Design review of the part built by this model. Coordinates are the model's own, in mm. A direction names the side the tool comes from. Coordinates: 2 decimals unless noted, no trailing zeros. Write each loop counter-clockwise with the first axis right and the second up, starting at its lowest first coordinate (ties: lowest second). Pieces come first, ordered by that corner, then holes. Notation, with made-up numbers: (54, 10.25) - (74, 10.25) arc R20 cw to (74, 18.25) - close; hole circle Ø7 at (-16.75, 26.25). An arc over 180 degrees is marked (long way). Answer as CSV lines item,"result". Start each with the question number.
Q1. We need section B-B (y = 2.4). Write out the cut boundary in (x, z).
Q2. We need section A-A (x = -6.35). Write out the cut boundary in (y, z) (3 decimals), plus the area to 3 significant figures.
Q3. Mouldability with a two-part tool opening along X and no side actions: class faces 5 (the face through (0, 2, -8)), 6 (the face through (52.003, 1.565, -51.522)), 7 (the face through (22, 2, -6.537)) as pulls with the +X half, pulls with the -X half, needs draft (parallel to the pull), parting line crosses it, or undercut.
Q4. For line 1 along Z through (x, y) = (50.8, 2.3); line 2 along X through (y, z) = (2.1, -50); line 3 along Z through (x, y) = (48, 0.7), list the stretches that pass through material, from the lowest coordinate up. Write a range as [from, to].
Q5. We need section C-C (z = -36). Write out the cut boundary in (x, y) (3 decimals), plus the area to 3 significant figures.
Q6. Machinability: for faces 1 (the face through (44.45, 2, -9)), 2 (the face through (54, 2, -29.464)), 3 (the face through (-9, 2, -10.414)), 4 (the face through (0, 2, -35)), which of the approach directions +Z, -Z, +X, -X, +Y, -Y give a long, thin tool a straight path to every point of the face, cutting with its end or side? Answer none if there is none.
Q7. Clearance check with flat-ended pins moving along their axes: pin 1 (2 mm diameter, centred on x = 50.8, z = -50.419, fed in from +Y); pin 2 (1 mm diameter, centred on x = 56, y = 1.5, fed in from +Z); pin 3 (8 mm diameter, centred on x = 39, z = -22.5, fed in from -Y); pin 4 (1 mm diameter, centred on y = 1.5, z = -37.5, fed in from -X). State where each tip first meets the part, or that it passes through.
from build123d import *

# Parameters (mm, degrees)
BOSS_EXTRUDE1_DEPTH   = 3.175
F_4_CLEARANCE_HOLE1_D = 3.2639
SKETCH6_W             = 47.36250333
SKETCH6_H             = 20.126599321
CUT_EXTRUDE2_DEPTH    = 95.829208522
SKETCH8_W             = 57.220052793
SKETCH8_H             = 21.750209978
CUT_EXTRUDE4_DEPTH    = 88.381999067


with BuildPart() as part:
    # Sketch2 → Boss-Extrude1 (new body)
    with BuildSketch(Plane(origin=(0, 0, 0), x_dir=(1, 0, 0), z_dir=(0, 1, 0))):
        Polygon((0, 40.894), (-19.05, 40.894), (-19.05, 59.944), (0, 59.944), (0, 70.358), (44.45, 70.358), (44.45, 59.944), (63.5, 59.944), (63.5, 40.894), (44.45, 40.894), (44.45, 29.464), (63.5, 29.464), (63.5, 10.414), (44.45, 10.414), (44.45, 0), (0, 0), (0, 10.414), (-19.05, 10.414), (-19.05, 29.464), (0, 29.464), align=None)
    extrude(amount=BOSS_EXTRUDE1_DEPTH)

    # #4 Clearance Hole1 (through all)
    with Locations(Plane(origin=(0, 3.175, 0), x_dir=(1, 0, 0), z_dir=(0, 1, 0))):
        with Locations((-6.35, 50.419), (50.8, 50.419), (50.8, 19.939), (-6.35, 19.939)):
            Hole(F_4_CLEARANCE_HOLE1_D / 2)

    # Sketch6 → Cut-Extrude2 (cut, through all)
    with BuildSketch(Plane.XZ):
        with Locations((20.768748335, -70.00729966)):
            Rectangle(SKETCH6_W, SKETCH6_H)
    extrude(amount=-CUT_EXTRUDE2_DEPTH, mode=Mode.SUBTRACT)

    # Sketch8 → Cut-Extrude4 (cut, through all)
    with BuildSketch(Plane.XZ):
        with Locations((24.07463768, 4.33828372)):
            Rectangle(SKETCH8_W, SKETCH8_H)
    extrude(amount=-CUT_EXTRUDE4_DEPTH, mode=Mode.SUBTRACT)


solid = part.part
Results list:
1,outline,"(-19.05, -59.94) - (63.5, -59.94) - (63.5, -40.89) - (44.45, -40.89) - (44.45, -29.46) - (63.5, -29.46) - (63.5, -10.41) - (44.45, -10.41) - (44.45, -6.54) - (0, -6.54) - (0, -10.41) - (-19.05, -10.41) - (-19.05, -29.46) - (0, -29.46) - (0, -40.89) - (-19.05, -40.89) - close; hole circle Ø3.26 at (-6.35, -50.42); hole circle Ø3.26 at (-6.35, -19.94); hole circle Ø3.26 at (50.8, -50.42); hole circle Ø3.26 at (50.8, -19.94)"
2,outline,"(0, -59.944) - (3.175, -59.944) - (3.175, -52.051) - (0, -52.051) - close; (0, -48.787) - (3.175, -48.787) - (3.175, -40.894) - (0, -40.894) - close; (0, -29.464) - (3.175, -29.464) - (3.175, -21.571) - (0, -21.571) - close; (0, -18.307) - (3.175, -18.307) - (3.175, -10.414) - (0, -10.414) - close"
2,area,"100 mm2"
3,face 5,"pulls with the -X half"
3,face 6,"undercut"
3,face 7,"needs draft"
4,line 1,"z = [-59.94, -52.05], [-48.79, -40.89], [-29.46, -21.57], [-18.31, -10.41]"
4,line 2,"x = [-19.05, -7.93], [-4.77, 49.22], [52.38, 63.5]"
4,line 3,"z = [-59.94, -40.89], [-29.46, -10.41]"
5,outline,"(0, 0) - (44.45, 0) - (44.45, 3.175) - (0, 3.175) - close"
5,area,"141 mm2"
6,face 1,"+Z, +X, +Y, -Y"
6,face 2,"+X, +Y, -Y"
6,face 3,"+Z, -X, +Y, -Y"
6,face 4,"-X, +Y, -Y"
7,pin 1,"passes through"
7,pin 2,"stops at z = -10.41"
7,pin 3,"stops at y = 0"
7,pin 4,"stops at x = 0"
